Geometry: final body of the model. Coordinates: model frame, mm. Face numbers are marked on the shaded views. A direction names the side the tool comes from. Give positions to 0.01 mm unless a question says otherwise; leave off trailing zeros. Loops run counter-clockwise (first coordinate to the right, second up) from the corner with the lowest first, then second, coordinate; pieces in that order, holes last. Notation, with made-up numbers: (24.5, 71) - (35.5, 71) arc R21 cw to (35.5, 93) - close; hole circle Ø7 at (-23.5, -0.5). An arc over 180 degrees is marked (long way). Use one line per item in the form item = value.
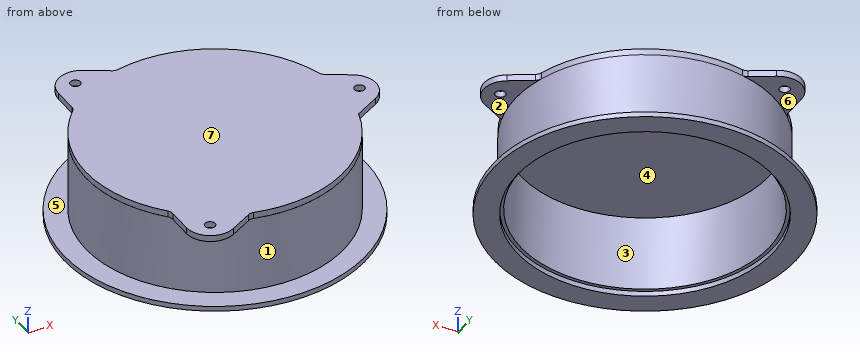
```python
from build123d import *

# Parameters (mm, degrees)
SKETCH4_R      = 151.840016695
SKETCH4_R_2    = 128.375867971
EXTRUDE1_DEPTH = 5.08
SKETCH6_R      = 129.999844579
SKETCH6_R_2    = 124.85482448
EXTRUDE2_DEPTH = 76.2
SKETCH8_R      = 5.099609744
EXTRUDE3_DEPTH = 6.35


with BuildPart() as part:
    # Sketch4 → Extrude1 (new body)
    with BuildSketch(Plane.XY):
        Circle(SKETCH4_R)
        Circle(SKETCH4_R_2, mode=Mode.SUBTRACT)
    extrude(amount=EXTRUDE1_DEPTH)

    # Sketch6 → Extrude2 (add)
    with BuildSketch(Plane.XY.offset(5.08)):
        with Locations(Location((0, 0, 0), (0, 0, 180))):
            Circle(SKETCH6_R)
        with Locations(Location((0, 0, 0), (0, 0, 180))):
            Circle(SKETCH6_R_2, mode=Mode.SUBTRACT)
    extrude(amount=EXTRUDE2_DEPTH)

    # Sketch8 → Extrude3 (add)
    with BuildSketch(Plane.XY.offset(81.28)):
        with BuildLine():
            Line((-92.869363805, -93.93198337), (-92.869363805, -119.06007059))
            ThreePointArc((-92.869363805, -119.06007059), (-80.804363805, -139.957263584), (-56.674363805, -139.957263584))
            Line((-56.674363805, -139.957263584), (-34.912801923, -127.393219973))
            ThreePointArc((-34.912801923, -127.393219973), (-32.224618976, -126.455362905), (-29.379828181, -126.569681633))
            ThreePointArc((-29.379828181, -126.569681633), (66.249521237, -111.776829211), (125.135094286, -34.989524014))
            Line((125.135094286, -34.989524014), (149.54372761, -20.897192993))
            ThreePointArc((149.54372761, -20.897192993), (161.60872761, 0), (149.54372761, 20.897192993))
            Line((149.54372761, 20.897192993), (127.782165728, 33.461236604))
            ThreePointArc((127.782165728, 33.461236604), (125.625866209, 35.320342792), (124.302473734, 37.841163253))
            ThreePointArc((124.302473734, 37.841163253), (64.96741224, 112.526858836), (-29.379828181, 126.569681633))
            ThreePointArc((-29.379828181, 126.569681633), (-32.224618976, 126.455362905), (-34.912801923, 127.393219973))
            Line((-34.912801923, 127.393219973), (-56.674363805, 139.957263584))
            ThreePointArc((-56.674363805, 139.957263584), (-80.804363805, 139.957263584), (-92.869363805, 119.06007059))
            Line((-92.869363805, 119.06007059), (-92.869363805, 93.93198337))
            ThreePointArc((-92.869363805, 93.93198337), (-93.401247233, 91.135020113), (-94.922645552, 88.72851838))
            ThreePointArc((-94.922645552, 88.72851838), (-129.93482448, 0), (-94.922645552, -88.72851838))
            ThreePointArc((-94.922645552, -88.72851838), (-93.401247233, -91.135020113), (-92.869363805, -93.93198337))
        make_face()
        with Locations((-72.432875103, 125.457419816)):
            Circle(SKETCH8_R, mode=Mode.SUBTRACT)
        with Locations((144.865750205, 0)):
            Circle(SKETCH8_R, mode=Mode.SUBTRACT)
        with Locations((-72.432875103, -125.457419816)):
            Circle(SKETCH8_R, mode=Mode.SUBTRACT)
    extrude(amount=EXTRUDE3_DEPTH)


solid = part.part
```
(1) Cut plane B-B (x = 0). Return the cut outline in (y, z), plus the area to 3 significant figures.
Solution:
outline = (-151.84, 0) - (-128.38, 0) - (-128.38, 5.08) - (-124.85, 5.08) - (-124.85, 81.28) - (124.85, 81.28) - (124.85, 5.08) - (128.38, 5.08) - (128.38, 0) - (151.84, 0) - (151.84, 5.08) - (130, 5.08) - (130, 81.28) - (129.93, 81.28) - (129.93, 87.63) - (-129.93, 87.63) - (-129.93, 81.28) - (-130, 81.28) - (-130, 5.08) - (-151.84, 5.08) - close
area = 2,670 mm2
(2) Cut plane C-C (z = 17). Return the cut outline in (x, y).
Solution:
outline = circle Ø260 at (0, 0); hole circle Ø249.71 at (0, 0)
(3) Cut plane D-D (y = 114.5). Return the cut outline in (x, z).
Solution:
outline = (-99.73, 0) - (-58.05, 0) - (-58.05, 5.08) - (-49.78, 5.08) - (-49.78, 81.28) - (49.78, 81.28) - (49.78, 5.08) - (58.05, 5.08) - (58.05, 0) - (99.73, 0) - (99.73, 5.08) - (61.56, 5.08) - (61.56, 81.28) - (61.42, 81.28) - (61.42, 87.63) - (-92.87, 87.63) - (-92.87, 81.28) - (-61.56, 81.28) - (-61.56, 5.08) - (-99.73, 5.08) - close
(4) Material intervals for L1, parallel to Y at x = 0, z = 56; L2, parallel to Z at x = -57, y = -66.5; L3, parallel to Y at x = 37.5, z = 4.5, sorted ascending. Write a range as from..to.
Solution:
L1 = -130..-124.85, 124.85..130
L2 = 81.28..87.63
L3 = -147.14..-122.78, 122.78..147.14
(5) Pull-direction query (X, two-part tool) for the marked faces 1, 2, 3 and 4; classes: released by +X, released by -X, zero draft, split by the parting line, or undercut.
Solution:
face_1 = split by the parting line
face_2 = zero draft
face_3 = undercut
face_4 = undercut
(6) Pin query (flat end, axial travel): P1, Ø5, axis at x = 38.5, z = 78.5, coming from the -Y side; P2, Ø3, axis at x = -59.5, y = 75.5, coming from the -Z side; P3, Ø5, axis at y = -111, z = 84.5, coming from the -X side. Return the tip coordinate at first contact, or that it passes through.
Solution:
P1 = -124.92
P2 = 81.28
P3 = -92.87
(7) Access query for the marked faces 5, 6 and 7. Directions: +Z, -Z, +X, -X, +Y, -Y. A direction counts if a zero-diameter tool reaches every point of the face in a straight line with its end or side. Return the directions, or none.
Solution:
face_5 = none
face_6 = -X, +Y
face_7 = +Z, +X, -X, +Y, -Y
(8) Cut plane A-A (y = 0). Return the cut outline in (x, z), plus the area to 3 significant figures.
Solution:
outline = (-151.84, 0) - (-128.38, 0) - (-128.38, 5.08) - (-124.85, 5.08) - (-124.85, 81.28) - (124.85, 81.28) - (124.85, 5.08) - (128.38, 5.08) - (128.38, 0) - (151.84, 0) - (151.84, 5.08) - (130, 5.08) - (130, 81.28) - (139.77, 81.28) - (139.77, 87.63) - (-129.93, 87.63) - (-129.93, 81.28) - (-130, 81.28) - (-130, 5.08) - (-151.84, 5.08) - close; (149.97, 81.28) - (161.61, 81.28) - (161.61, 87.63) - (149.97, 87.63) - close
area = 2,810 mm2
